Design review of the part built by this model. Coordinates are the model's own, in mm. Face numbers are marked on the shaded views. A direction names the side the tool comes from. Give positions to 0.01 mm unless a question says otherwise; leave off trailing zeros. Write each loop counter-clockwise with the first axis right and the second up, starting at its lowest first coordinate (ties: lowest second). Pieces come first, ordered by that corner, then holes. Notation, with made-up numbers: M 66.25,33.25 L 104.25,33.25 A22 cw 104.25,58.25 Z; hole C 86,39.5 d7. An arc over 180 degrees is marked long. Use a Markdown table: item, result. Add a question column.
```python
from build123d import *

# Parameters (mm, degrees)
SKETCH1_W           = 25
SKETCH1_H           = 23.5
BOSS_EXTRUDE1_DEPTH = 1
SKETCH2_R           = 1
CUT_EXTRUDE1_DEPTH  = 1
SKETCH3_W           = 9
SKETCH3_H           = 5
BOSS_EXTRUDE2_DEPTH = 1
SKETCH4_W           = 5
SKETCH4_H           = 4.5
BOSS_EXTRUDE3_DEPTH = 0.9
SKETCH5_W           = 8
SKETCH5_H           = 8
BOSS_EXTRUDE4_DEPTH = 4
SKETCH6_R           = 3.5
BOSS_EXTRUDE5_DEPTH = 1
SKETCH8_W           = 21
SKETCH8_H           = 5
BOSS_EXTRUDE6_DEPTH = 2


with BuildPart() as part:
    # Sketch1 → Boss-Extrude1 (new body)
    with BuildSketch(Plane(origin=(0, 0, 0), x_dir=(1, 0, 0), z_dir=(0, 1, 0))):
        Rectangle(SKETCH1_W, SKETCH1_H)
    extrude(amount=BOSS_EXTRUDE1_DEPTH)

    # Sketch2 → Cut-Extrude1 (cut)
    with BuildSketch(Plane(origin=(0, 1, 0), x_dir=(1, 0, 0), z_dir=(0, 1, 0))):
        with Locations((-10.5, 9.75)):
            Circle(SKETCH2_R)
        with Locations((10.5, 9.75)):
            Circle(SKETCH2_R)
        with Locations((10.5, -3.25)):
            Circle(SKETCH2_R)
        with Locations((-10.5, -3.25)):
            Circle(SKETCH2_R)
    extrude(amount=-CUT_EXTRUDE1_DEPTH, mode=Mode.SUBTRACT)

    # Sketch3 → Boss-Extrude2 (add)
    with BuildSketch(Plane(origin=(0, 1, 0), x_dir=(1, 0, 0), z_dir=(0, 1, 0))):
        with Locations((0, 8.25)):
            Rectangle(SKETCH3_W, SKETCH3_H)
    extrude(amount=BOSS_EXTRUDE2_DEPTH)

    # Sketch4 → Boss-Extrude3 (add)
    with BuildSketch(Plane(origin=(0, 1, 0), x_dir=(1, 0, 0), z_dir=(0, 1, 0))):
        with Locations((0, 3.5)):
            Rectangle(SKETCH4_W, SKETCH4_H)
    extrude(amount=BOSS_EXTRUDE3_DEPTH)

    # Sketch5 → Boss-Extrude4 (add)
    with BuildSketch(Plane(origin=(0, 1, 0), x_dir=(1, 0, 0), z_dir=(0, 1, 0))):
        with Locations((0, -2.75)):
            Rectangle(SKETCH5_W, SKETCH5_H)
    extrude(amount=BOSS_EXTRUDE4_DEPTH)

    # Sketch6 → Boss-Extrude5 (add)
    with BuildSketch(Plane(origin=(0, 5, 0), x_dir=(1, 0, 0), z_dir=(0, 1, 0))):
        with Locations((0, -2.75)):
            Circle(SKETCH6_R)
    extrude(amount=BOSS_EXTRUDE5_DEPTH)

    # Sketch8 → Boss-Extrude6 (add)
    with BuildSketch(Plane.XZ):
        with Locations((0, 9.24)):
            Rectangle(SKETCH8_W, SKETCH8_H)
    extrude(amount=BOSS_EXTRUDE6_DEPTH)


solid = part.part
```
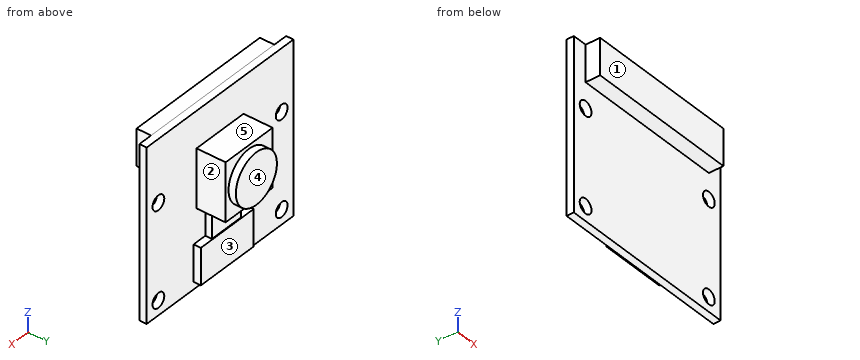
(1) For pin 1 (1.5 mm diameter, centred on x = -5, z = -6.5, fed in from -Y); pin 2 (3 mm diameter, centred on y = 4, z = 4, fed in from -X); pin 3 (4.5 mm diameter, centred on x = -1.5, y = 3.5, fed in from +Z), all flat-tipped, find the tip position at first contact; note any pin that passes through.
(2) Wall thickness on L1, parallel to X at y = 0.2, z = -9.75; L2, parallel to Z at x = -10.5, y = 0.6; L3, parallel to X at y = 0.5, z = 3.75: over which ranges is each line inside the solid? List them lowest first.
(3) Add section D-D on y = 5.5. Give the boundary of the cut face in (x, z).
(4) Add section A-A on z = -9.75. Give the boundary of the cut face in (x, y).
(5) Add section B-B on z = 7.5. Give the boundary of the cut face in (x, y), then the cut area to 3 significant figures.
(6) Machinability: for the marked faces 1, 2, 3, 4 and 5, which of the approach directions +Z, -Z, +X, -X, +Y, -Y give a long, thin tool a straight path to every point of the face, cutting with its end or side? Answer none if there is none.
From the geometry:
| question | item | result |
|---|---|---|
| 1 | pin 1 | stops at y = 0 |
| 1 | pin 2 | stops at x = -4 |
| 1 | pin 3 | stops at z = 6.75 |
| 2 | L1 | x = -12.5 to -11.5, -9.5 to 9.5, 11.5 to 12.5 |
| 2 | L2 | z = -11.75 to -10.75, -8.75 to 2.25, 4.25 to 11.75 |
| 2 | L3 | x = -12.5 to -11.37, -9.63 to 9.63, 11.37 to 12.5 |
| 3 | outline | C 0,2.75 d7 |
| 4 | outline | M -12.5,0 L -11.5,0 L -11.5,1 L -12.5,1 Z; M -9.5,0 L 9.5,0 L 9.5,1 L 4.5,1 L 4.5,2 L -4.5,2 L -4.5,1 L -9.5,1 Z; M 11.5,0 L 12.5,0 L 12.5,1 L 11.5,1 Z |
| 5 | outline | M -12.5,0 L -10.5,0 L -10.5,-2 L 10.5,-2 L 10.5,0 L 12.5,0 L 12.5,1 L -12.5,1 Z |
| 5 | area | 67.0 mm^2 |
| 6 | face 1 | +Z, -Z, +X, -X, -Y |
| 6 | face 2 | +Z, +X, +Y |
| 6 | face 3 | -Z, +X, -X, +Y |
| 6 | face 4 | +Z, -Z, +X, -X, +Y |
| 6 | face 5 | +Z, +X, -X, +Y |
